```python
from build123d import *

# Parameters (mm, degrees)
SKETCH1_W              = 203.2
SKETCH1_H              = 152.4
MAIN_BODY_DEPTH        = 9.525
SKETCH2_W              = 177.8
SKETCH2_H              = 127
SLIDE_INSET_DEPTH      = 6.35
F_10_32_TAPPED_HOLE2_D = 4.826


with BuildPart() as part:
    # Sketch1 → main body (new body)
    with BuildSketch(Plane(origin=(0, 0, 0), x_dir=(1, 0, 0), z_dir=(0, 1, 0))):
        with Locations((173.045515995, -23.140372536)):
            Rectangle(SKETCH1_W, SKETCH1_H)
    extrude(amount=MAIN_BODY_DEPTH)

    # Sketch2 → slide inset (cut)
    with BuildSketch(Plane(origin=(0, 9.525, 0), x_dir=(1, 0, 0), z_dir=(0, 1, 0))):
        with Locations((173.045515995, -23.140372536)):
            Rectangle(SKETCH2_W, SKETCH2_H)
    extrude(amount=-SLIDE_INSET_DEPTH, mode=Mode.SUBTRACT)

    # Sweep for sealing ribs: sweep along a path in gasket bump profiles
    with BuildLine(Plane(origin=(0, 9.525, 0), x_dir=(1, 0, 0), z_dir=(0, 1, 0))) as sweep_for_sealing_ribs_path:
        Line((79.065515995, 40.359627464), (79.065515995, -86.640372536))
        ThreePointArc((79.065515995, -86.640372536), (80.553413547, -90.232474985), (84.145515995, -91.720372536))
        Line((84.145515995, -91.720372536), (261.945515995, -91.720372536))
        ThreePointArc((261.945515995, -91.720372536), (265.537618444, -90.232474985), (267.025515995, -86.640372536))
        Line((267.025515995, -86.640372536), (267.025515995, 40.359627464))
        ThreePointArc((267.025515995, 40.359627464), (265.537618444, 43.951729912), (261.945515995, 45.439627464))
        Line((261.945515995, 45.439627464), (84.145515995, 45.439627464))
        ThreePointArc((84.145515995, 45.439627464), (80.553413547, 43.951729912), (79.065515995, 40.359627464))
    # gasket bump shape → Sweep for sealing ribs (sweep)
    with BuildSketch(Plane(origin=(0, 0, 23.140372536), x_dir=(-1, 0, 0), z_dir=(0, 0, -1))):
        with BuildLine():
            Line((-77.795515995, 9.525), (-80.335515995, 9.525))
            ThreePointArc((-80.335515995, 9.525), (-79.065515995, 10.31875), (-77.795515995, 9.525))
        make_face()
        with BuildLine():
            Line((-76.525515995, 9.525), (-73.985515995, 9.525))
            ThreePointArc((-73.985515995, 9.525), (-75.255515995, 10.033), (-76.525515995, 9.525))
        make_face()
    sweep(path=sweep_for_sealing_ribs_path.line)

    # #10-32 Tapped Hole2 (through all)
    with Locations(Plane.XZ):
        with Locations((173.045515995, 23.140372536)):
            Hole(F_10_32_TAPPED_HOLE2_D / 2)


solid = part.part
```
For this review, take the finished solid that the model builds, in its own axes (mm). A direction names the side the tool comes from. Give positions to 0.01 mm unless a question says otherwise; leave off trailing zeros. Loops run counter-clockwise (first coordinate to the right, second up) from the corner with the lowest first, then second, coordinate; pieces in that order, holes last. Notation, with made-up numbers: M 67,46 L 88,46 A25 cw 88,72 Z; hole C 50,-18 d6. An arc over 180 degrees is marked long. One line per item, written item: value. Start each with the question number.
Q1. Add section A-A (y = 7.75). Give the boundary of the cut face in (x, z).
Q2. Clearance check with flat-ended pins moving along their axes: pin 1 Ø12 at (x, z) = (152, 27) entering from +Y (3 decimals); pin 2 Ø6 at (x, z) = (223.5, -30.5) entering from -Y. State where each tip first meets the part, or that it passes through.
Q3. Add section C-C (z = 52). Give the boundary of the cut face in (x, y) (1 decimal).
Q4. Add section B-B (x = 114). Give the boundary of the cut face in (y, z) (1 decimal), and give its area (3 significant figures).
Q5. For L1, parallel to Z at x = 179.5, y = 9; L2, parallel to X at y = 6.5, z = -32; L3, parallel to Z at x = 95, y = 9.75, list the stretches that pass through material, from the lowest coordinate up.
Q6. Machinability: for faces 1 (the face through (172, 5, -53.06)), 2 (the face through (172, 6, 86.64)), which of the approach directions +Z, -Z, +X, -X, +Y, -Y give a long, thin tool a straight path to every point of the face, cutting with its end or side? Answer none if there is none.
Q7. Draft analysis for pull direction Z (two halves, no side actions). For faces 3 (the face through (84.146, 6, 24)), 4 (the face through (172, 3.175, 8)), 5 (the face through (172, 5, 99.34)), 6 (the face through (71.446, 5, 24)), state which applies: released by +Z, released by -Z, zero draft, split by the parting line, or undercut.
Reply:
1. outline: M 71.45,-53.06 L 274.65,-53.06 L 274.65,99.34 L 71.45,99.34 Z; hole M 84.15,-40.36 L 261.95,-40.36 L 261.95,86.64 L 84.15,86.64 Z
2. pin 1: y = 3.175
2. pin 2: y = 0
3. outline: M 71.4,0 L 274.6,0 L 274.6,9.5 L 272.1,9.5 A1.8 ccw 269.6,9.5 L 268.3,9.5 A1.4 ccw 265.8,9.5 L 261.9,9.5 L 261.9,3.2 L 84.1,3.2 L 84.1,9.5 L 80.3,9.5 A1.4 ccw 77.8,9.5 L 76.5,9.5 A1.8 ccw 74,9.5 L 71.4,9.5 Z
4. outline: M 0,-53.1 L 9.5,-53.1 L 9.5,-50.5 A1.8 ccw 9.5,-48 L 9.5,-46.7 A1.4 ccw 9.5,-44.2 L 9.5,-40.4 L 3.2,-40.4 L 3.2,86.6 L 9.5,86.6 L 9.5,90.5 A1.4 ccw 9.5,93 L 9.5,94.3 A1.8 ccw 9.5,96.8 L 9.5,99.3 L 0,99.3 Z
4. area: 650 mm²
5. L1: -53.06 to -40.36, 86.64 to 99.34
5. L2: 71.45 to 84.15, 261.95 to 274.65
5. L3: -50.23 to -48.27, -46.57 to -44.31, 90.59 to 92.85, 94.55 to 96.51
6. face 1: -Z, +X, -X, +Y, -Y
6. face 2: +Y
7. face 3: undercut
7. face 4: undercut
7. face 5: released by +Z
7. face 6: zero draft
